```python
from build123d import *

# Parameters (mm, degrees)
PAD_DEPTH    = 4
SKETCH001_W  = 2.45
SKETCH001_H  = 4.3
PAD001_DEPTH = 5
PAD002_DEPTH = 23
PAD003_DEPTH = 10


with BuildPart() as part:
    # Sketch → Pad (new body)
    with BuildSketch(Plane.XZ):
        Polygon((0, 0), (4.8, 0), (4.8, 0.9), (3.8, 0.9), (3.8, 3.1), (5.8, 3.1), (5.8, 7.4), (0, 7.4), align=None)
    pad = extrude(amount=PAD_DEPTH)

    # Sketch001 → Pad001 (join)
    with BuildSketch(Plane.XZ.offset(4)):
        with Locations((4.575, 5.25)):
            Rectangle(SKETCH001_W, SKETCH001_H)
    pad001 = extrude(amount=PAD001_DEPTH)

    # Sketch002 → Pad002 (join)
    with BuildSketch(Plane.XZ.offset(9)):
        Polygon((5.8, 7.4), (0, 7.4), (0, 5.4), (3.35, 5.4), (3.35, 3.1), (5.8, 3.1), align=None)
    pad002 = extrude(amount=PAD002_DEPTH)

    # Sketch003 → Pad003 (join)
    with BuildSketch(Plane.XZ.offset(32)):
        Polygon((4.8, 0), (4.8, 0.9), (3.8, 0.9), (3.8, 3.1), (5.8, 3.1), (5.8, 7.4), (0, 7.4), (0, 5.4), (2.2, 5.4), (2.2, 0), align=None)
    pad003 = extrude(amount=PAD003_DEPTH)

    # Mirrored: Pad, Pad001, Pad002, Pad003 across Sketch V_Axis
    add(pad.mirror(Plane(origin=(0, 0, 0), x_dir=(0, -1, 0), z_dir=(1, 0, 0))))
    add(pad001.mirror(Plane(origin=(0, 0, 0), x_dir=(0, -1, 0), z_dir=(1, 0, 0))))
    add(pad002.mirror(Plane(origin=(0, 0, 0), x_dir=(0, -1, 0), z_dir=(1, 0, 0))))
    add(pad003.mirror(Plane(origin=(0, 0, 0), x_dir=(0, -1, 0), z_dir=(1, 0, 0))))


solid = part.part
```
Read the model definition and answer for the solid it produces. Units are mm, in the model's axes. A direction names the side the tool comes from. Round coordinates to 2 decimals unless told otherwise and drop trailing zeros. Loops run counter-clockwise (first coordinate to the right, second up) from the corner with the lowest first, then second, coordinate; pieces in that order, holes last. Notation, with made-up numbers: (-15, 33) -> (23, 33) arc R25 ccw to (23, 60) -> close; hole circle Ø5 at (89.5, -5.5). An arc over 180 degrees is marked (long way). One line per item, written item: value.
1) A cutting plane is placed at C-C (x = 0). Determine the outline of the cut face in (y, z).
Answer list:
outline: (-42, 5.4) -> (-9, 5.4) -> (-9, 7.4) -> (-42, 7.4) -> close; (-4, 0) -> (0, 0) -> (0, 7.4) -> (-4, 7.4) -> close
2) A cutting plane is placed at D-D (y = -26). Determine the outline of the cut face in (x, z).
Answer list:
outline: (-5.8, 3.1) -> (-3.35, 3.1) -> (-3.35, 5.4) -> (3.35, 5.4) -> (3.35, 3.1) -> (5.8, 3.1) -> (5.8, 7.4) -> (-5.8, 7.4) -> close
3) Flat-ended cylindrical pins translate along their axes: P1, Ø1.5, axis at x = 2, y = -12, coming from the -Z side; P2, Ø0.7, axis at y = -35.5, z = 2.5, coming from the +X side; P3, Ø1, axis at y = -38, z = 0.5, coming from the -X side; P4, Ø2, axis at y = -24, z = 1.5, coming from the +X side. Find the tip coordinate at first contact, or state that the pin passes through.
Answer list:
P1: stops at z = 5.4
P2: stops at x = 3.8
P3: stops at x = -4.8
P4: passes through
4) Consider L1, parallel to X at y = -38, z = 3.75; L2, parallel to Y at x = 1.75, z = 6.5; L3, parallel to X at y = -28, z = 5. Determine where each line is inside the solid, lowest interval first. Write a range as [from, to].
Answer list:
L1: x = [-5.8, -2.2], [2.2, 5.8]
L2: y = [-42, -9], [-4, 0]
L3: x = [-5.8, -3.35], [3.35, 5.8]
5) A cutting plane is placed at A-A (y = -4.5). Determine the outline of the cut face in (x, z), and give its area (3 significant figures).
Answer list:
outline: (-5.8, 3.1) -> (-3.35, 3.1) -> (-3.35, 7.4) -> (-5.8, 7.4) -> close; (3.35, 3.1) -> (5.8, 3.1) -> (5.8, 7.4) -> (3.35, 7.4) -> close
area: 21.1 mm²
6) For faces 1 (the face through (-3, -32, 2)), 2 (the face through (-4, -2, 0.9)), 3 (the face through (3.8, -37, 2)), 4 (the face through (-4.8, -2, 0.4)), determine the directions among +Z, -Z, +X, -X, +Y, -Y from which every point of the face is accessible in a straight line to the end or side of a thin tool.
Answer list:
face 1: -Z
face 2: -X, +Y, -Y
face 3: +X, +Y, -Y
face 4: -Z, -X, +Y, -Y
7) The mould has two halves that part along X. Classify faces 5 (the face through (-3.8, -2, 2)), 6 (the face through (0, 0, 4)), 7 (the face through (0, -9, 6)): pulls with the +X half, pulls with the -X half, needs draft (parallel to the pull), parting line crosses it, or undercut.
Answer list:
face 5: pulls with the -X half
face 6: needs draft
face 7: undercut
8) A cutting plane is placed at B-B (z = 1.75). Determine the outline of the cut face in (x, y), and give its area (3 significant figures).
Answer list:
outline: (-3.8, -42) -> (-2.2, -42) -> (-2.2, -32) -> (-3.8, -32) -> close; (-3.8, -4) -> (3.8, -4) -> (3.8, 0) -> (-3.8, 0) -> close; (2.2, -42) -> (3.8, -42) -> (3.8, -32) -> (2.2, -32) -> close
area: 62.4 mm²
